```python
from build123d import *

# Parameters (mm, degrees)
SKETCH3_R          = 2.25
CUT_EXTRUDE2_DEPTH = 34.35416016


with BuildPart() as part:
    # Sketch1 → Revolve1 (revolve)
    with BuildSketch(Plane(origin=(0, 0, 0), x_dir=(0, 0, -1), z_dir=(1, 0, 0)), mode=Mode.PRIVATE) as revolve1_sk:
        with BuildLine():
            Line((0, 0), (0, -22.5))
            ThreePointArc((0, -22.5), (-3.535533906, -21.035533906), (-5, -17.5))
            Line((-5, -17.5), (-5, -12))
            Line((-5, -12), (-3, -12))
            Line((-3, -12), (-3, -6))
            Line((-3, -6), (-5, -6))
            Line((-5, -6), (-5, 0))
            Line((-5, 0), (0, 0))
        make_face()
    revolve1 = revolve(revolve1_sk.sketch.rotate(Axis((0, 0, 5), (0, 0, -1)), 270), axis=Axis((0, 0, 5), (0, 0, -1)))

    # Mirror1: Revolve1 across plane
    add(revolve1.mirror(Plane.XY))

    # Sketch3 → Cut-Extrude2 (cut, through all)
    with BuildSketch(Plane(origin=(0, 0, -5), x_dir=(-1, 0, 0), z_dir=(0, 0, -1))):
        Circle(SKETCH3_R)
    extrude(amount=-CUT_EXTRUDE2_DEPTH, mode=Mode.SUBTRACT)


solid = part.part
```
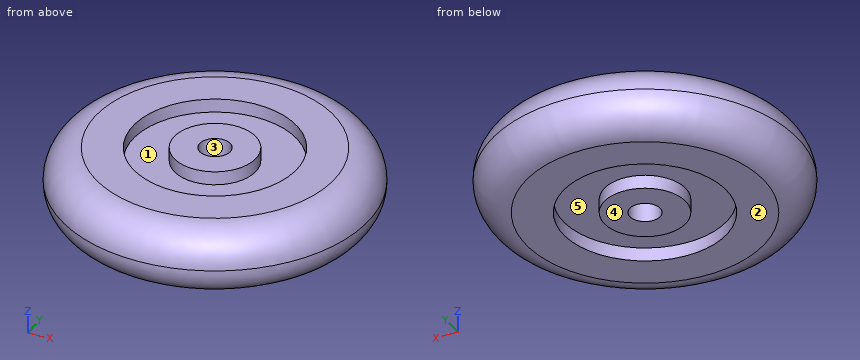
Design review of the part built by this model. Coordinates are the model's own, in mm. Face numbers are marked on the shaded views. A direction names the side the tool comes from. Coordinates: 2 decimals unless noted, no trailing zeros. Loops run counter-clockwise (first coordinate to the right, second up) from the corner with the lowest first, then second, coordinate; pieces in that order, holes last. Notation, with made-up numbers: (-21, 70) - (24, 70) arc R12 ccw to (24, 83) - close; hole circle Ø8 at (78, 45.25). An arc over 180 degrees is marked (long way). Use CSV: the item, a comma, the result in double quotes. Start each with the question number.
1) Consider section A-A on z = -1.75. Write out the cut boundary in (x, y), then the cut area to 3 significant figures.
2) For pin 1 Ø1.5 at (x, y) = (6.5, 1.5) entering from +Z; pin 2 Ø1 at (x, z) = (-4, 2) entering from -Y; pin 3 Ø1.5 at (x, z) = (-3, 2) entering from -Y; pin 4 Ø6 at (x, z) = (0, -1) entering from -Y, all flat-tipped, find the tip position at first contact; note any pin that passes through.
3) Wall thickness on L1, parallel to Y at x = 0, z = 3.7; L2, parallel to Y at x = 0, z = 3.25; L3, parallel to Y at x = 0, z = 2: over which ranges is each line inside the solid? List them lowest first. Write a range as from..to.
4) The part is to be moulded in two halves that separate along X. For the marked faces 3, 4 and 5, say which applies: +X half, -X half, draft (parallel to the pull), parting line (faces both ways), or undercut.
5) Tool access review of the marked faces 1 and 2: name each direction out of +Z, -Z, +X, -X, +Y, -Y from which nothing blocks a thin tool from reaching the whole face with its end or side.
Geometry says:
1,outline,"circle Ø44.37 at (0, 0); hole circle Ø4.5 at (0, 0)"
1,area,"1,530 mm^2"
2,pin 1,"z = 5"
2,pin 2,"y = -21.93"
2,pin 3,"y = -22.16"
2,pin 4,"y = -22.5"
3,L1,"-20.86..-12, -6..-2.25, 2.25..6, 12..20.86"
3,L2,"-21.3..-12, -6..-2.25, 2.25..6, 12..21.3"
3,L3,"-22.08..-2.25, 2.25..22.08"
4,face 3,"undercut"
4,face 4,"draft"
4,face 5,"undercut"
5,face 1,"+Z"
5,face 2,"-Z, +X, -X, +Y, -Y"
